Autodesk Fusion 360 part; units mm, degrees
sketch "Sketch1" plane through (0, 0, 0) normal (0, 1, 0) x (1, 0, 0)
  line L0 (-5, 29.899) -> (-5, -40.101)
  line L1 (5, -40.101) -> (5, 29.899)
  circle A0 centre (0, -45) radius 1.55
  arc A1 (-5, -40.101) -> (5, -40.101) centre (0, -45) ccw
  arc A2 (5, 29.899) -> (-5, 29.899) centre (0, 34.798) ccw
  circle A3 centre (0, 34.798) radius 1.55
  dimension "d3" = 3.1
  dimension "d4" = 14
  dimension "d7" = 70
  dimension "d8" = 7
  dimension "d9" = 3.1
extrude "Extrude1" add sketch "Sketch1" along normal blind 5
sketch "Sketch2" plane through (0, 0, 0) normal (0, -1, 0) x (1, 0, 0)
  circle A0 centre (0, -34.798) radius 1.55
  circle A1 centre (0, 45) radius 1.55
  arc A2 (-5, -29.899) -> (5, -29.899) centre (0, -34.798) ccw
  line L0 (5, -29.899) -> (5, 40.101)
  arc A3 (5, 40.101) -> (-5, 40.101) centre (0, 45) ccw
  line L1 (-5, 40.101) -> (-5, -29.899)
extrude "Extrude2" cut sketch "Sketch2" against normal blind 1
extrude "Extrude3" cut 1 faces at (-1.6667, 1, 16.7677) along direction (0, 1, 0) blind 0.4
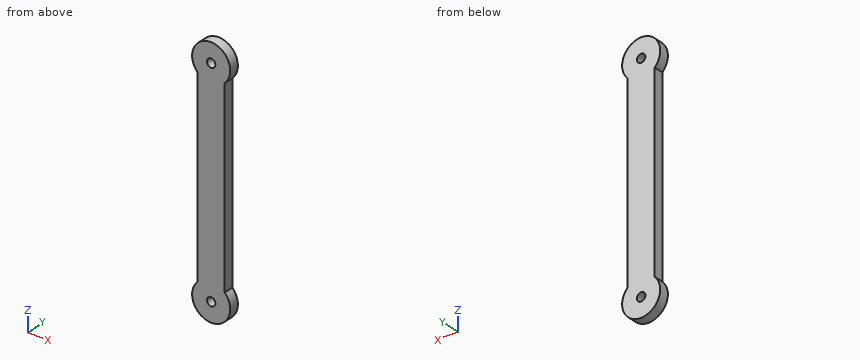
CAD build for the part. Positions are in the model's coordinates, mm. Coordinates: 2 decimals unless noted, no trailing zeros. Loops run counter-clockwise (first coordinate to the right, second up) from the corner with the lowest first, then second, coordinate; pieces in that order, holes last. Notation, with made-up numbers: (0.5, 4) - (41.5, 4) arc R29 cw to (41.5, 33) - close; hole circle Ø11 at (47.25, -28). An arc over 180 degrees is marked (long way). Return JSON: item names as keys, results as strings.
1. Drop flat-ended pins along their axis: pin 1 (1 mm diameter, centred on y = 4, z = 33, fed in from +X); pin 2 (1.5 mm diameter, centred on x = 2.5, y = 2.5, fed in from -Z). Give the stop position or say it passes through.
Result:
{"pin 1": "stops at x = 5", "pin 2": "stops at z = -41.58"}
2. Band-saw the part on A-A (x = 0). Give the cut face in (y, z).
Result:
{"outline": "(1.4, -41.8) - (5, -41.8) - (5, -36.35) - (1.4, -36.35) - close; (1.4, -33.25) - (5, -33.25) - (5, 43.45) - (1.4, 43.45) - close; (1.4, 46.55) - (5, 46.55) - (5, 52) - (1.4, 52) - close"}
3. Probe L1, parallel to Z at x = 0, y = 2.9; L2, parallel to X at y = 2.7, z = 45; L3, parallel to Z at x = 0.5, y = 3.75. List the from-to ranges inside material, lowest first. Write a range as from..to.
Result:
{"L1": "z = -41.8..-36.35, -33.25..43.45, 46.55..52", "L2": "x = -7..-1.55, 1.55..7", "L3": "z = -41.78..-36.27, -33.33..43.53, 46.47..51.98"}
4. Band-saw the part on B-B (z = 45). Give the cut face in (x, y).
Result:
{"outline": "(-7, 1.4) - (-1.55, 1.4) - (-1.55, 5) - (-7, 5) - close; (1.55, 1.4) - (7, 1.4) - (7, 5) - (1.55, 5) - close"}
5. Band-saw the part on D-D (z = -20). Give the cut face in (x, y), and give its area (3 significant figures).
Result:
{"outline": "(-5, 1.4) - (5, 1.4) - (5, 5) - (-5, 5) - close", "area": "36.0 mm2"}
6. Band-saw the part on C-C (y = 2.6). Give the cut face in (x, z).
Result:
{"outline": "(-5, -29.9) arc R7 ccw (long way) to (5, -29.9) - (5, 40.1) arc R7 ccw (long way) to (-5, 40.1) - close; hole circle Ø3.1 at (0, -34.8); hole circle Ø3.1 at (0, 45)"}
